```python
from build123d import *

# Parameters (mm, degrees)
BELT_PULLEY_W       = 6.35
BELT_PULLEY_H       = 6.35
BOSS_EXTRUDE1_DEPTH = 6.35


with BuildPart() as part:
    # Belt Pulley → Boss-Extrude1 (new body)
    with BuildSketch(Plane(origin=(0, 0, 0), x_dir=(1, 0, 0), z_dir=(0, 1, 0))):
        with BuildLine():
            Line((1.26, 12.637341493), (0, 12.7))
            ThreePointArc((0, 12.7), (-0.016303366, 12.699989535), (-0.032606705, 12.699958142))
            Line((-0.032606705, 12.699958142), (-0.41408034, 13.288550052))
            Line((-0.41408034, 13.288550052), (-3.23677354, 12.894972743))
            Line((-3.23677354, 12.894972743), (-3.390219288, 12.239134495))
            Line((-3.390219288, 12.239134495), (-4.587769161, 11.842397313))
            ThreePointArc((-4.587769161, 11.842397313), (-4.602967816, 11.8364981), (-4.618158887, 11.830579381))
            Line((-4.618158887, 11.830579381), (-5.18649638, 12.24162082))
            Line((-5.18649638, 12.24162082), (-7.676402878, 10.854946515))
            Line((-7.676402878, 10.854946515), (-7.582570675, 10.187964564))
            Line((-7.582570675, 10.187964564), (-8.555934674, 9.385413249))
            ThreePointArc((-8.555934674, 9.385413249), (-8.567975957, 9.374422009), (-8.58000312, 9.36341532))
            Line((-8.58000312, 9.36341532), (-9.258447344, 9.541392864))
            Line((-9.258447344, 9.541392864), (-11.079291471, 7.348899611))
            Line((-11.079291471, 7.348899611), (-10.750853876, 6.760853565))
            Line((-10.750853876, 6.760853565), (-11.3685738, 5.660877118))
            ThreePointArc((-11.3685738, 5.660877118), (-11.375831468, 5.646278279), (-11.383070389, 5.631670135))
            Line((-11.383070389, 5.631670135), (-12.079993691, 5.55254693))
            Line((-12.079993691, 5.55254693), (-12.985860359, 2.850343093))
            Line((-12.985860359, 2.850343093), (-12.467174689, 2.42065183))
            Line((-12.467174689, 2.42065183), (-12.645824039, 1.171808165))
            ThreePointArc((-12.645824039, 1.171808165), (-12.647317904, 1.155573381), (-12.648790926, 1.139336692))
            Line((-12.648790926, 1.139336692), (-13.270069953, 0.813798767))
            Line((-13.270069953, 0.813798767), (-13.138616847, -2.033168055))
            Line((-13.138616847, -2.033168055), (-12.499734477, -2.246472349))
            Line((-12.499734477, -2.246472349), (-12.215185668, -3.475519974))
            ThreePointArc((-12.215185668, -3.475519974), (-12.210713975, -3.491198106), (-12.20622216, -3.506870484))
            Line((-12.20622216, -3.506870484), (-12.667949736, -4.03485743))
            Line((-12.667949736, -4.03485743), (-11.516930327, -6.64208859))
            Line((-11.516930327, -6.64208859), (-10.84413586, -6.610197989))
            Line((-10.84413586, -6.610197989), (-10.134818786, -7.653459882))
            ThreePointArc((-10.134818786, -7.653459882), (-10.124985463, -7.666463943), (-10.115135453, -7.679455369))
            Line((-10.115135453, -7.679455369), (-10.354952711, -8.338583773))
            Line((-10.354952711, -8.338583773), (-8.339818549, -10.353958256))
            Line((-8.339818549, -10.353958256), (-7.723976606, -10.081179762))
            Line((-7.723976606, -10.081179762), (-6.685688469, -10.797757624))
            ThreePointArc((-6.685688469, -10.797757624), (-6.671821559, -10.806331343), (-6.657943654, -10.814887253))
            Line((-6.657943654, -10.814887253), (-6.643461944, -11.516138172))
            Line((-6.643461944, -11.516138172), (-4.036368063, -12.667468487))
            Line((-4.036368063, -12.667468487), (-3.560651511, -12.190642346))
            Line((-3.560651511, -12.190642346), (-2.333618876, -12.483758366))
            ThreePointArc((-2.333618876, -12.483758366), (-2.317591183, -12.486743815), (-2.301559671, -12.489708687))
            Line((-2.301559671, -12.489708687), (-2.034734829, -13.138374297))
            Line((-2.034734829, -13.138374297), (0.812216296, -13.270166905))
            Line((0.812216296, -13.270166905), (1.0835593, -12.653691131))
            Line((1.0835593, -12.653691131), (2.333618876, -12.483758366))
            ThreePointArc((2.333618876, -12.483758366), (2.349642724, -12.480752344), (2.365662699, -12.477725754))
            Line((2.365662699, -12.477725754), (2.8487945, -12.986200172))
            Line((2.8487945, -12.986200172), (5.551106344, -12.08065575))
            Line((5.551106344, -12.08065575), (5.581429424, -11.407788812))
            Line((5.581429424, -11.407788812), (6.685688469, -10.797757624))
            ThreePointArc((6.685688469, -10.797757624), (6.699544361, -10.78916611), (6.713389212, -10.780556817))
            Line((6.713389212, -10.780556817), (7.347578346, -11.080167754))
            Line((7.347578346, -11.080167754), (9.54028872, -9.259585095))
            Line((9.54028872, -9.259585095), (9.325496576, -8.621201402))
            Line((9.325496576, -8.621201402), (10.134818786, -7.653459882))
            ThreePointArc((10.134818786, -7.653459882), (10.144635409, -7.640443209), (10.154435313, -7.627413944))
            Line((10.154435313, -7.627413944), (10.854031022, -7.677697283))
            Line((10.854031022, -7.677697283), (12.24100224, -5.187956164))
            Line((12.24100224, -5.187956164), (11.810103742, -4.67027297))
            Line((11.810103742, -4.67027297), (12.215185668, -3.475519974))
            ThreePointArc((12.215185668, -3.475519974), (12.219637231, -3.459836115), (12.224068656, -3.444146554))
            Line((12.224068656, -3.444146554), (12.894586664, -3.238311251))
            Line((12.894586664, -3.238311251), (13.288500578, -0.415665006))
            Line((13.288500578, -0.415665006), (12.699690955, -0.088598295))
            Line((12.699690955, -0.088598295), (12.645824039, 1.171808165))
            ThreePointArc((12.645824039, 1.171808165), (12.644309334, 1.188041018), (12.642773792, 1.204271914))
            Line((12.642773792, 1.204271914), (13.193656926, 1.638426659))
            Line((13.193656926, 1.638426659), (12.541313278, 4.412764015))
            Line((12.541313278, 4.412764015), (11.874114533, 4.505042071))
            Line((11.874114533, 4.505042071), (11.3685738, 5.660877118))
            ThreePointArc((11.3685738, 5.660877118), (11.361297397, 5.675466629), (11.354002271, 5.690046786))
            Line((11.354002271, 5.690046786), (11.710850711, 6.293885971))
            Line((11.710850711, 6.293885971), (10.100352127, 8.645224804))
            Line((10.100352127, 8.645224804), (9.444873147, 8.490251542))
            Line((9.444873147, 8.490251542), (8.555934674, 9.385413249))
            ThreePointArc((8.555934674, 9.385413249), (8.543879292, 9.396389022), (8.531809829, 9.40734931))
            Line((8.531809829, 9.40734931), (8.646429216, 10.099321106))
            Line((8.646429216, 10.099321106), (6.295282453, 11.710100078))
            Line((6.295282453, 11.710100078), (5.740049306, 11.328805496))
            Line((5.740049306, 11.328805496), (4.587769161, 11.842397313))
            ThreePointArc((4.587769161, 11.842397313), (4.572562944, 11.848277011), (4.557349193, 11.854137182))
            Line((4.557349193, 11.854137182), (4.414259544, 12.540786964))
            Line((4.414259544, 12.540786964), (1.64, 13.193461449))
            Line((1.64, 13.193461449), (1.26, 12.637341493))
        make_face()
        Rectangle(BELT_PULLEY_W, BELT_PULLEY_H, mode=Mode.SUBTRACT)
    extrude(amount=BOSS_EXTRUDE1_DEPTH)


solid = part.part
```
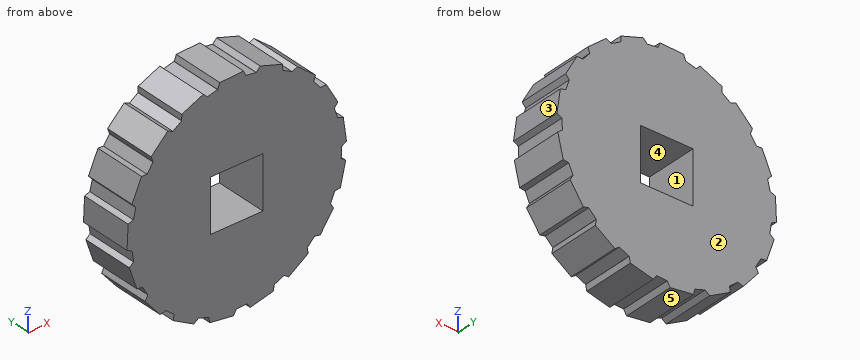
Input: part model. Units: mm. Frame: model coordinates. Face numbers are marked on the shaded views. A direction names the side the tool comes from. Give positions to 0.01 mm unless a question says otherwise; leave off trailing zeros. Order: outer loops, then holes, each group sorted by start corner. A loop starts at its lowest first (then second) coordinate and runs counter-clockwise, first axis right, second up. Notation, with made-up numbers: (54.25, 89.5) -> (107.25, 89.5) arc R22 cw to (107.25, 108.5) -> close; hole circle Ø5 at (-8, 16.5). An arc over 180 degrees is marked (long way). Write each question's results on one line, items separated by ' | '. Start each with the question number.
Item 1: Set-up query: the marked faces 1 and 2. Return all of +Z, -Z, +X, -X, +Y, -Y with unobstructed straight access to the full face (end or side cutting, diameter ignored); none if empty.
Item 2: Mould query, pull axis X, two halves, no side actions, for the marked faces 3, 4 and 5. Classes: pulls with the +X half, pulls with the -X half, needs draft (parallel to the pull), parting line crosses it, or undercut.
Item 3: Cut plane A-A on z = -5. Return the cut outline in (x, y), then the cut area to 3 significant figures.
Item 4: Contact query for flat-ended pins moving along their axis: P1, Ø3, axis at y = 1, z = -6.5, coming from the +X side; P2, Ø2, axis at x = -3.5, y = 4, coming from the -Z side; P3, Ø3, axis at x = -1, y = 3, coming from the +Z side. Output: stop coordinate, or through.
Item 5: Cut plane B-B on x = -6. Return the cut outline in (y, z), then the cut area to 3 significant figures.
Item 6: Line query: line 1 (X direction, y = 1, z = 5); line 2 (Z direction, x = -0.5, y = 4) (3 decimals); line 3 (X direction, y = 4.25, z = 11.5). Output: solid intervals per line, ascending.
Established:
1) face 1: +Y, -Y | face 2: +Z, -Z, +X, -X, +Y
2) face 3: pulls with the +X half | face 4: undercut | face 5: pulls with the -X half
3) outline: (-12.27, 0) -> (11.66, 0) -> (11.66, 6.35) -> (-12.27, 6.35) -> close | area: 152 mm^2
4) P1: x = 11.71 | P2: z = -13 | P3: z = 13.26
5) outline: (0, -11.79) -> (6.35, -11.79) -> (6.35, 11.8) -> (0, 11.8) -> close | area: 150 mm^2
6) line 1: -12.24 to 12.08 | line 2: -13.277 to -3.175, 3.175 to 13.209 | line 3: -6.64 to 5.58
